The listing builds one solid part. Answer for the finished solid, in the listing's coordinates (mm). A direction names the side the tool comes from. Give positions to 0.01 mm unless a question says otherwise; leave off trailing zeros. Write each loop counter-clockwise with the first axis right and the second up, starting at its lowest first coordinate (ties: lowest second). Pieces come first, ordered by that corner, then holes. Notation, with made-up numbers: (71.25, 88.5) - (102.25, 88.5) arc R11 cw to (102.25, 106.5) - close; hole circle Ø10 at (-8, 0). An arc over 180 degrees is marked (long way). Answer in a Markdown table with one row per item. Add a question column.
from build123d import *

# Parameters (mm, degrees)
BASE_FLANGE1_DEPTH                        = 1193.8
CUT_EXTRUDE1_DEPTH                        = 1198.055003958
F_1_4_CLEARANCE_HOLE1_D                   = 6.7564
F_10_0_1935_DIAMETER_HOLE1_D              = 4.9149
HOLE_FOR_1_4_SELF_CLINCHING_NUTS_S_SS_C_D = 8.7376
FILLET1_R                                 = 2.54


# Sheet-metal steps are written as plain solids
with BuildPart() as part:
    # Sketch1 → Base-Flange1 (new body)
    with BuildSketch(Plane.XY):
        with BuildLine():
            Line((-38.1, 44.45), (-38.1, 5.76326))
            ThreePointArc((-38.1, 5.76326), (-36.411980228, 1.688019772), (-32.33674, 0))
            Line((-32.33674, 0), (32.33674, 0))
            ThreePointArc((32.33674, 0), (36.411980228, 1.688019772), (38.1, 5.76326))
            Line((38.1, 5.76326), (38.1, 44.45))
            Line((38.1, 44.45), (35.51174, 44.45))
            Line((35.51174, 44.45), (35.51174, 5.76326))
            ThreePointArc((35.51174, 5.76326), (34.58180403, 3.51819597), (32.33674, 2.58826))
            Line((32.33674, 2.58826), (-32.33674, 2.58826))
            ThreePointArc((-32.33674, 2.58826), (-34.58180403, 3.51819597), (-35.51174, 5.76326))
            Line((-35.51174, 5.76326), (-35.51174, 44.45))
            Line((-35.51174, 44.45), (-38.1, 44.45))
        make_face()
    extrude(amount=BASE_FLANGE1_DEPTH)

    # Sketch6 → Cut-Extrude1 (cut, through all)
    with BuildSketch(Plane(origin=(38.1, 0, 0), x_dir=(0, 0, -1), z_dir=(1, 0, 0))):
        Polygon((-1140.478324087, 44.45), (-1193.8, 30.1625), (-1193.8, 44.45), align=None)
        Polygon((0, 44.45), (-53.321675913, 44.45), (0, 30.1625), align=None)
    extrude(amount=-CUT_EXTRUDE1_DEPTH, mode=Mode.SUBTRACT)

    # 1/4 Clearance Hole1 (through all)
    with Locations(Plane.ZY.offset(38.1)):
        with Locations((1181.1, 22.225), (12.7, 22.225)):
            Hole(F_1_4_CLEARANCE_HOLE1_D / 2)

    # #10 (0.1935) Diameter Hole1 (through all)
    with Locations(Plane(origin=(38.1, 0, 0), x_dir=(0, 0, -1), z_dir=(1, 0, 0))):
        with Locations((-619.125, 34.925), (-619.125, 12.7), (-574.675, 12.7), (-574.675, 34.925), (-1146.175, 12.7), (-1104.9, 34.925), (-1054.1, 34.925), (-1146.175, 34.925), (-47.625, 34.925), (-139.7, 34.925), (-88.9, 34.925), (-47.625, 12.7)):
            Hole(F_10_0_1935_DIAMETER_HOLE1_D / 2)

    # Hole for 1/4 Self-clinching Nuts (S,SS,CLS,CLSS)1 (through all)
    with Locations(Plane(origin=(38.1, 0, 0), x_dir=(0, 0, -1), z_dir=(1, 0, 0))):
        with Locations((-711.2, 31.75), (-482.6, 31.75)):
            Hole(HOLE_FOR_1_4_SELF_CLINCHING_NUTS_S_SS_C_D / 2)

    # Fillet1
    fillet1_edges = [part.edges().sort_by_distance(p)[0] for p in [
        (36.80587, 30.1625, 1193.8),
        (36.80587, 44.45, 1140.478324087),
        (-36.80587, 30.1625, 0),
        (-36.80587, 44.45, 53.321675913),
        (36.80587, 44.45, 53.321675913),
        (36.80587, 30.1625, 0),
        (-36.80587, 44.45, 1140.478324087),
        (-36.80587, 30.1625, 1193.8),
    ]]
    fillet(fillet1_edges, radius=FILLET1_R)


solid = part.part
1. Straight lines are drawn through the part: L1, parallel to X at y = 10.5, z = 99.5; L2, parallel to Z at x = 37, y = 12; L3, parallel to Y at x = -37.1, z = 711.2. For each, find the intervals that lie inside material, in ascending order. Write a range as [from, to].
2. Section B-B (x = -20.5) is taken. Give the vertices of the cut face in (y, z), and give its area (3 significant figures).
3. A tool of negligible diameter and unlimited length cuts with its end or side. For faces 4 (the face through (0, 2, 1193.8)), 5 (the face through (0, 2.588, 589)), from which of +Z, -Z, +X, -X, +Y, -Y can it reach the whole face along a straight path? Write none if from no direction.
4. The mould has two halves that part along X. Classify faces 1 (the face through (-38.1, 25, 589)), 2 (the face through (0, 0, 589)), 3 (the face through (-35.512, 25, 589)): +X half, -X half, draft (parallel to the pull), parting line (faces both ways), or undercut.
5. Given pin 1 Ø4.5 at (y, z) = (34.925, 1146.175) entering from +X, flat-ended and moving along its own axis, determine where the tip first touches the part or whether it passes through.
6. Section A-A (z = 512) is taken. Give the vertices of the cut face in (x, y) (3 decimals), and give its area (3 significant figures).
Geometry check:
| question | item | result |
|---|---|---|
| 1 | L1 | [-38.1, -35.51], [35.51, 38.1] |
| 1 | L2 | [0, 45.27], [49.98, 572.32], [577.03, 616.77], [621.48, 1143.82], [1148.53, 1193.8] |
| 1 | L3 | [2.52, 27.38], [36.12, 44.45] |
| 2 | outline | (0, 0) - (2.59, 0) - (2.59, 1193.8) - (0, 1193.8) - close |
| 2 | area | 3,090 mm² |
| 3 | face 4 | +Z, +X, -X, +Y, -Y |
| 3 | face 5 | +Z, -Z, +Y |
| 4 | face 1 | -X half |
| 4 | face 2 | draft |
| 4 | face 3 | undercut |
| 5 | pin 1 | through |
| 6 | outline | (-38.1, 5.763) arc R5.763 ccw to (-32.337, 0) - (32.337, 0) arc R5.763 ccw to (38.1, 5.763) - (38.1, 44.45) - (35.512, 44.45) - (35.512, 5.763) arc R3.175 cw to (32.337, 2.588) - (-32.337, 2.588) arc R3.175 cw to (-35.512, 5.763) - (-35.512, 44.45) - (-38.1, 44.45) - close |
| 6 | area | 404 mm² |
